Read the model definition and answer for the solid it produces. Units are mm, in the model's axes. A direction names the side the tool comes from. Coordinates: 2 decimals unless noted, no trailing zeros. Loops run counter-clockwise (first coordinate to the right, second up) from the corner with the lowest first, then second, coordinate; pieces in that order, holes last. Notation, with made-up numbers: M 32.5,-36 L 81.5,-36 A27 ccw 81.5,0 Z; hole C 3,59.25 d5. An arc over 180 degrees is marked long. One line per item, written item: value. Start each with the question number.
1. For faces 4 (the face through (12.5, 18, -49)), 5 (the face through (13, 25, 14.5)), 6 (the face through (25, 46, 0)), 7 (the face through (19, 25, 7.5)), determine the directions among +Z, -Z, +X, -X, +Y, -Y from which every point of the face is accessible in a straight line to the end or side of a thin tool.
2. The part is cut by section C-C (x = 40.5). Write down the section's boundary in (y, z), then the cut area to 3 significant figures.
3. Consider probe 1 along Y at (x, z) = (33.5, 10.5); probe 2 along Y at (x, z) = (34, 10); probe 3 along Y at (x, z) = (27.5, -27.5). Determine where each line is inside the solid, lowest interval first.
4. Flat-ended cylindrical pins translate along their axes: pin 1 (6 mm diameter, centred on x = 54, y = 38.5, fed in from +Z); pin 2 (9.5 mm diameter, centred on y = 21, z = 19.5, fed in from -X); pin 3 (10 mm diameter, centred on x = 12, y = 24.5, fed in from +Z); pin 4 (6 mm diameter, centred on x = 40.5, y = 18.5, fed in from +Z). Find the tip coordinate at first contact, or state that the pin passes through.
5. The part is cut by section D-D (y = 6.5). Write down the section's boundary in (x, z).
6. The part is cut by section B-B (z = -27.5). Write down the section's boundary in (x, y).
7. The part is cut by section A-A (y = 29.85). Write down the section's boundary in (x, z), then the cut area to 3 significant figures.
8. Determine the mould class of faces 1 (the face through (24.82, 12.59, -92.15)), 2 (the face through (44, 18, 0)), 3 (the face through (25, 5, -95)) for opening direction Y: +Y half, -Y half, draft (parallel to the pull), parting line (faces both ways), or undercut.
Autodesk Inventor part; units mm, degrees
ref_plane "YZ Plane" through (0, 0, 0) normal (1, 0, 0) x (0, 1, 0)
ref_plane "XZ Plane" through (0, 0, 0) normal (0, 1, 0) x (-1, 0, 0)
ref_plane "XY Plane" through (0, 0, 0) normal (0, 0, 1) x (1, 0, 0)
sketch "Sketch1" plane through (0, 0, 0) normal (0, 0, 1) x (1, 0, 0)
  line L0 (0, 0) -> (50, 0)
  line L1 (50, 0) -> (50, 50)
  line L2 (50, 50) -> (0, 50)
  line L3 (0, 50) -> (0, 0)
  dimension "d0" = 50
  dimension "d1" = 50
extrude "Extrusion1" add sketch "Sketch1" along normal blind 32
sketch "Sketch2" plane through (0, 0, 32) normal (0, 0, 1) x (1, 0, 0)
  line L0 (50, 0) -> (50, 50)
  line L1 (50, 15) -> (9, 15)
  line L2 (9, 15) -> (9, 35)
  line L3 (9, 35) -> (50, 35)
  line L4 (50, 35) -> (50, 15)
  line L5 (0, 0) -> (50, 0)
  point P0 (50, 35)
  dimension "d4" = 41
  dimension "d5" = 20
  dimension "d6" = 15
extrude "Extrusion2" cut sketch "Sketch2" against normal blind 17.5
sketch "Sketch3" plane through (0, 0, 0) normal (-1, 0, 0) x (0, 0, 1)
  line L0 (32, 50) -> (32, 0)
  line L1 (32, 35) -> (10.5, 35) construction
  line L2 (32, 35) -> (53.5, 35) construction
  line L3 (10.5, 35) -> (10.5, 15) construction
  line L4 (10.5, 15) -> (32, 15) construction
  line L5 (0, 50) -> (32, 50)
  line L6 (32, 29.85) -> (10.5, 29.85) construction
  line L7 (32, 20.15) -> (10.5, 20.15) construction
  point P0 (0, 0)
  dimension "d9" = 21.5
  dimension "d10" = 180
  dimension "d11" = 20
  dimension "d12" = 15
  dimension "d13" = 5.15
  dimension "d14" = 5.15
hole "Hole1" at (0, 29.85, 10.5) at (0, 20.15, 10.5) direction (1, 0, 0) diameter 4.3 end through all
sketch "Sketch4" plane through (0, 0, 14.5) normal (0, 0, 1) x (1, 0, 0)
  line L0 (9, 35) -> (50, 35)
  line L1 (50, 15) -> (9, 15)
  line L2 (18, 35) -> (20.4, 35)
  line L3 (20.4, 35) -> (20.4, 15)
  line L4 (20.4, 15) -> (18, 15)
  line L5 (18, 15) -> (18, 35)
  line L6 (9, 15) -> (9, 35)
  point P0 (0, 0)
  point P1 (18, 15)
  dimension "d22" = 9
  dimension "d23" = 2.4
extrude "Extrusion3" cut sketch "Sketch4" against normal blind 7 contours L0 L3 L1 L5
chamfer "Chamfer1" distance 5 angle 45 4 edges at (0, 50, 16) (50, 50, 16) (0, 0, 16) (50, 0, 16)
sketch "Sketch7" plane through (0, 0, 14.5) normal (0, 0, 1) x (1, 0, 0)
  line L0 (18, 15) -> (18, 35)
  line L1 (18, 24.5) -> (16, 24.5)
  line L2 (16, 24.5) -> (16, 25.5)
  line L3 (16, 25.5) -> (18, 25.5)
  line L4 (18, 25.5) -> (18, 24.5)
  line L5 (9, 35) -> (50, 35)
  point P0 (0, 0)
  dimension "d45" = 2
  dimension "d46" = 1
  dimension "d47" = 9.5
extrude "Extrusion5" cut sketch "Sketch7" against normal blind 7
chamfer "Chamfer3" distance 7 distance2 2 1 edges at (16, 25, 7.5) measured on face at (16, 25.1667, 12.1667)
sketch "Sketch9" plane through (0, 0, 0) normal (0, 0, -1) x (-1, 0, 0)
  line L0 (-45, 50) -> (-5, 50)
  line L1 (-25, 50) -> (-25, 0) construction
  line L2 (-5, 0) -> (-45, 0)
  line L3 (-37.5, 0) -> (-37.5, 42.5)
  line L4 (-37.5, 42.5) -> (-12.5, 42.5)
  line L5 (-12.5, 42.5) -> (-12.5, 0)
  point P0 (0, 0)
  dimension "d61" = 42.5
  dimension "d62" = 25
  dimension "d63" = 12.5
extrude "Extrusion6" add sketch "Sketch9" along normal blind 100
sketch "Sketch10" plane through (12.5, 0, 0) normal (-1, 0, 0) x (0, 0, 1)
  line L0 (-100, 42.5) -> (-100, 0)
  line L1 (-100, 42.5) -> (0, 42.5)
  line L2 (0, 42.5) -> (0, 35)
  line L3 (0, 35) -> (-100, 35)
  line L4 (-100, 35) -> (-100, 42.5)
  point P0 (0, 0)
  dimension "d66" = 100
  dimension "d67" = 7.5
extrude "Extrusion7" add sketch "Sketch10" along normal blind 25 and the other way blind 50
chamfer "Chamfer4" distance 5 angle 45 4 edges at (-12.5, 38.75, 0) (-12.5, 38.75, -100) (62.5, 38.75, 0) (62.5, 38.75, -100)
chamfer "Chamfer5" distance 10 angle 45 1 edges at (25, 0, -100)
sketch "Sketch11" plane through (12.5, 0, 0) normal (-1, 0, 0) x (0, 0, 1)
  line L0 (-100, 10) -> (-100, 35)
  line L1 (-100, 12.5) -> (0, 12.5) construction
  line L2 (0, 0) -> (-90, 0)
  line L3 (-27.5, 0) -> (-27.5, 35) construction
  line L4 (-90, 0) -> (-90, 35) construction
  line L5 (-95, 35) -> (-5, 35)
  line L6 (0, 35) -> (0, 5)
  circle A0 centre (-90, 12.5) radius 2.15
  circle A1 centre (-27.5, 12.5) radius 2.15
  dimension "d78" = 12.5
  dimension "d79" = 27.5
  dimension "d80" = 10
  dimension "d81" = 4.3
  dimension "d82" = 4.3
extrude "Extrusion8" cut sketch "Sketch11" against normal through all
properties part number "ES117_MP1"
Answer block:
1. face 4: -Z, -X, -Y
1. face 5: +Z, +X
1. face 6: -Z, +X, -X, +Y
1. face 7: +Z
2. outline: M 0,0 L 35,0 L 35,-100 L 42.5,-100 L 42.5,0 L 50,0 L 50,32 L 35,32 L 35,14.5 L 15,14.5 L 15,32 L 0,32 Z; hole C 20.15,10.5 d4.3; hole C 29.85,10.5 d4.3
2. area: 1,970 mm2
3. probe 1: y = 0 to 18, 22.3 to 27.7, 32 to 50
3. probe 2: y = 0 to 18.06, 22.24 to 27.76, 31.94 to 50
3. probe 3: y = 0 to 10.35, 14.65 to 42.5
4. pin 1: stops at z = 0
4. pin 2: stops at x = 0
4. pin 3: stops at z = 32
4. pin 4: stops at z = 14.5
5. outline: M 0,0 L 12.5,0 L 12.5,-96.5 L 37.5,-96.5 L 37.5,0 L 50,0 L 50,32 L 0,32 Z
6. outline: M -12.5,35 L 12.5,35 L 12.5,14.65 L 37.5,14.65 L 37.5,35 L 62.5,35 L 62.5,42.5 L -12.5,42.5 Z; M 12.5,0 L 37.5,0 L 37.5,10.35 L 12.5,10.35 Z
7. outline: M 0,0 L 12.5,0 L 12.5,-100 L 37.5,-100 L 37.5,0 L 50,0 L 50,8.35 L 20.4,8.35 L 20.4,7.5 L 18,7.5 L 18,8.35 L 0,8.35 Z; M 0,12.65 L 18,12.65 L 18,14.5 L 9,14.5 L 9,32 L 0,32 Z; M 20.4,12.65 L 50,12.65 L 50,14.5 L 20.4,14.5 Z
7. area: 3,160 mm2
8. face 1: undercut
8. face 2: draft
8. face 3: -Y half
